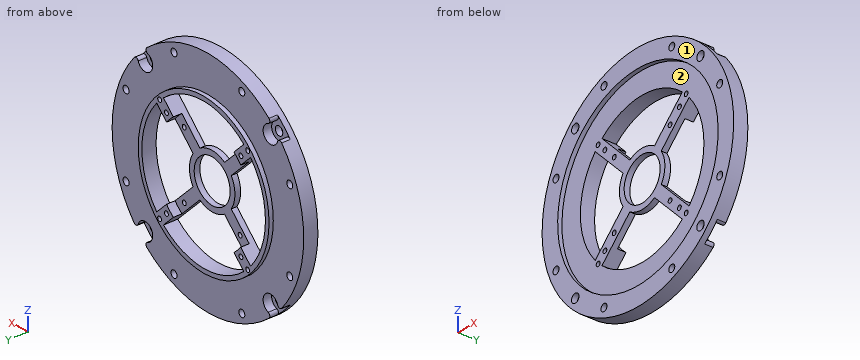
from build123d import *

# Parameters (mm, degrees)
SKETCH_1_R                       = 40
EXTRUDE_1_DEPTH                  = 5
CUT_EXTRUDE_1_DEPTH              = 57.789083458
CUT_EXTRUDE_1_DEPTH_BACK         = 1.5
SKETCH_2_R                       = 33.5
SKETCH_7_R                       = 27.3
EXTRUDE_3_DEPTH                  = 1.5
SKETCH_3_R                       = 25.8
CUT_EXTRUDE_2_DEPTH              = 57.940758688
EXTRUDE_2_DEPTH                  = 5
CUT_EXTRUDE_3_DEPTH              = 57.789083458
CUT_EXTRUDE_3_DEPTH_BACK         = 4
SKETCH_5_R                       = 7.515
CUT_EXTRUDE_4_DEPTH              = 57.835288334
CUT_EXTRUDE_4_DEPTH_BACK         = 57.835288334
SKETCH_6_R                       = 6.5
SKETCH_8_R                       = 20
SKETCH_8_R_2                     = 4.5
CUT_EXTRUDE_5_DEPTH              = 3
HOLE_WIZARD_M2_1_D               = 1.6
HOLE_WIZARD_M2_6_D               = 1.6
HOLE_WIZARD_M3_1_OUTLINE_R       = 1.25
HOLE_WIZARD_M3_1_DEPTH           = 5
SKETCH_25_R                      = 3.1
CUT_EXTRUDE_7_DEPTH              = 3
SKETCH_26_R                      = 1.55
CUT_EXTRUDE_8_DEPTH              = 57.747246629
FILLET_1_R                       = 1
PATTERN_CIRCULAR_1_COUNT         = 4
FILLET_1_OF_PATTERN_CIRCULAR_1_R = 1


# Read off the part's stored shape, not the designer's step: M3 螺纹孔1
with BuildPart() as part:
    # 草图1 → 凸台-拉伸1 (new body)
    with BuildSketch(Plane(origin=(0, 0, 0), x_dir=(1, 0, 0), z_dir=(0, 1, 0))):
        with Locations(Location((0, 0, 0), (0, 0, 270))):
            Circle(SKETCH_1_R)
    extrude(amount=EXTRUDE_1_DEPTH)

    # 草图2 → 切除-拉伸1 (cut, two sides: drawn at the far end of the back side and taken through both)
    with BuildSketch(Plane.XZ.offset(-CUT_EXTRUDE_1_DEPTH_BACK)):
        with Locations(Location((0, 0, 0), (0, 0, 90))):
            Circle(SKETCH_2_R)
    extrude(amount=CUT_EXTRUDE_1_DEPTH + CUT_EXTRUDE_1_DEPTH_BACK, mode=Mode.SUBTRACT)

    # 草图7 → 凸台-拉伸3 (add)
    with BuildSketch(Plane(origin=(0, 5, 0), x_dir=(1, 0, 0), z_dir=(0, 1, 0))):
        with Locations(Location((0, 0, 0), (0, 0, 270))):
            Circle(SKETCH_7_R)
    extrude(amount=EXTRUDE_3_DEPTH)

    # 草图3 → 切除-拉伸2 (cut, through all)
    with BuildSketch(Plane(origin=(0, 6.5, 0), x_dir=(1, 0, 0), z_dir=(0, 1, 0))):
        with Locations(Location((0, 0, 0), (0, 0, 270))):
            Circle(SKETCH_3_R)
    extrude(amount=-CUT_EXTRUDE_2_DEPTH, mode=Mode.SUBTRACT)

    # 草图4 → 凸台-拉伸2 (add)
    with BuildSketch(Plane.XZ.offset(-1.5)):
        with BuildLine():
            Line((-19.657568517, 16.829141392), (-7.981176331, 5.152749206))
            ThreePointArc((-7.981176331, 5.152749206), (-9.5, 0), (-7.981176331, -5.152749206))
            Line((-7.981176331, -5.152749206), (-19.657568517, -16.829141392))
            Line((-19.657568517, -16.829141392), (-16.829141392, -19.657568517))
            Line((-16.829141392, -19.657568517), (-5.152749206, -7.981176331))
            ThreePointArc((-5.152749206, -7.981176331), (0, -9.5), (5.152749206, -7.981176331))
            Line((5.152749206, -7.981176331), (16.829141392, -19.657568517))
            Line((16.829141392, -19.657568517), (19.657568517, -16.829141392))
            Line((19.657568517, -16.829141392), (7.981176331, -5.152749206))
            ThreePointArc((7.981176331, -5.152749206), (9.5, 0), (7.981176331, 5.152749206))
            Line((7.981176331, 5.152749206), (19.657568517, 16.829141392))
            Line((19.657568517, 16.829141392), (16.829141392, 19.657568517))
            Line((16.829141392, 19.657568517), (5.152749206, 7.981176331))
            ThreePointArc((5.152749206, 7.981176331), (0, 9.5), (-5.152749206, 7.981176331))
            Line((-5.152749206, 7.981176331), (-16.829141392, 19.657568517))
            Line((-16.829141392, 19.657568517), (-19.657568517, 16.829141392))
        make_face()
    extrude(amount=-EXTRUDE_2_DEPTH)

    # 草图5 → 切除-拉伸3 (cut, two sides: drawn at the far end of the back side and taken through both)
    with BuildSketch(Plane.XZ.offset(-1.5).offset(-CUT_EXTRUDE_3_DEPTH_BACK)):
        with Locations(Location((0, 0, 0), (0, 0, 270))):
            Circle(SKETCH_5_R)
    extrude(amount=CUT_EXTRUDE_3_DEPTH + CUT_EXTRUDE_3_DEPTH_BACK, mode=Mode.SUBTRACT)

    # 草图6 → 切除-拉伸4 (cut, two sides: drawn at the far end of the back side and taken through both)
    with BuildSketch(Plane.XZ.offset(-5.5).offset(-CUT_EXTRUDE_4_DEPTH_BACK)):
        with Locations(Location((0, 0, 0), (0, 0, 270))):
            Circle(SKETCH_6_R)
    extrude(amount=CUT_EXTRUDE_4_DEPTH + CUT_EXTRUDE_4_DEPTH_BACK, mode=Mode.SUBTRACT)

    # 草图8 → 切除-拉伸5 (cut)
    with BuildSketch(Plane(origin=(0, 6.5, 0), x_dir=(1, 0, 0), z_dir=(0, 1, 0))):
        Circle(SKETCH_8_R)
        Circle(SKETCH_8_R_2, mode=Mode.SUBTRACT)
    extrude(amount=-CUT_EXTRUDE_5_DEPTH, mode=Mode.SUBTRACT)

    # M2 螺纹孔1 (through all)
    with Locations(Plane(origin=(0, 3.5, 0), x_dir=(1, 0, 0), z_dir=(0, 1, 0))):
        with Locations((0, 0), (-11.66726189, 11.66726189), (11.66726189, 11.66726189), (11.66726189, -11.66726189), (-11.66726189, -11.66726189)):
            Hole(HOLE_WIZARD_M2_1_D / 2)

    # M2 螺纹孔6 (through all)
    with Locations(Plane(origin=(0, 6.5, 0), x_dir=(1, 0, 0), z_dir=(0, 1, 0))):
        with Locations((15.556349186, 15.556349186), (0, 0), (-15.556349186, 15.556349186), (-15.556349186, -15.556349186), (15.556349186, -15.556349186), (-18.384776311, 18.384776311), (18.384776311, 18.384776311), (18.384776311, -18.384776311), (-18.384776311, -18.384776311)):
            Hole(HOLE_WIZARD_M2_6_D / 2)

    # M3 螺纹孔1 outline → M3 螺纹孔1 (cut)
    with BuildSketch(Plane(origin=(0, 0, 0), x_dir=(1, 0, 0), z_dir=(0, 1, 0))):
        with Locations((34.183542703, 14.159286998)):
            Circle(HOLE_WIZARD_M3_1_OUTLINE_R)
        with Locations((34.183542703, -14.159286998)):
            Circle(HOLE_WIZARD_M3_1_OUTLINE_R)
        with Locations((14.159286998, -34.183542703)):
            Circle(HOLE_WIZARD_M3_1_OUTLINE_R)
        with Locations((-14.159286998, -34.183542703)):
            Circle(HOLE_WIZARD_M3_1_OUTLINE_R)
        with Locations((-34.183542703, -14.159286998)):
            Circle(HOLE_WIZARD_M3_1_OUTLINE_R)
        with Locations((-34.183542703, 14.159286998)):
            Circle(HOLE_WIZARD_M3_1_OUTLINE_R)
        with Locations((-14.159286998, 34.183542703)):
            Circle(HOLE_WIZARD_M3_1_OUTLINE_R)
        with Locations((14.159286998, 34.183542703)):
            Circle(HOLE_WIZARD_M3_1_OUTLINE_R)
    extrude(amount=HOLE_WIZARD_M3_1_DEPTH, mode=Mode.SUBTRACT)

    # 草图25 → 切除-拉伸7 (cut)
    with BuildSketch(Plane(origin=(0, 5, 0), x_dir=(1, 0, 0), z_dir=(0, 1, 0))):
        with Locations((-26.162950904, -26.162950904)):
            Circle(SKETCH_25_R)
    cut_extrude_7 = extrude(amount=-CUT_EXTRUDE_7_DEPTH, mode=Mode.SUBTRACT)

    # 草图26 → 切除-拉伸8 (cut, through all)
    with BuildSketch(Plane(origin=(0, 2, 0), x_dir=(1, 0, 0), z_dir=(0, 1, 0))):
        with Locations(Location((-26.162950904, -26.162950904, 0), (0, 0, 270))):
            Circle(SKETCH_26_R)
    cut_extrude_8 = extrude(amount=-CUT_EXTRUDE_8_DEPTH, mode=Mode.SUBTRACT)

    # 圆角1
    fillet_1_edges = [part.edges().sort_by_distance(p)[0] for p in [
        (-28.852633786, 3.5, 27.704251003),
        (-27.704251003, 3.5, 28.852633786),
    ]]
    fillet(fillet_1_edges, radius=FILLET_1_R)

    # 阵列(圆周)1: 切除-拉伸7, 切除-拉伸8 ×4 about axis
    pattern_circular_1_axis = Axis((0, 0, 0), (0, 1, 0))
    add([cut_extrude_7.rotate(pattern_circular_1_axis, i * 360 / PATTERN_CIRCULAR_1_COUNT) for i in range(1, PATTERN_CIRCULAR_1_COUNT)], mode=Mode.SUBTRACT)
    add([cut_extrude_8.rotate(pattern_circular_1_axis, i * 360 / PATTERN_CIRCULAR_1_COUNT) for i in range(1, PATTERN_CIRCULAR_1_COUNT)], mode=Mode.SUBTRACT)

    # 圆角1 of 阵列(圆周)1
    fillet_1_of_pattern_circular_1_edges = [part.edges().sort_by_distance(p)[0] for p in [
        (27.704251003, 3.5, 28.852633786),
        (28.852633786, 3.5, 27.704251003),
        (28.852633786, 3.5, -27.704251003),
        (27.704251003, 3.5, -28.852633786),
        (-27.704251003, 3.5, -28.852633786),
        (-28.852633786, 3.5, -27.704251003),
    ]]
    fillet(fillet_1_of_pattern_circular_1_edges, radius=FILLET_1_OF_PATTERN_CIRCULAR_1_R)


solid = part.part
Could you check a few things on this model? Use its own coordinates, in mm. Face numbers are marked on the shaded views. Give positions to 0.01 mm unless a question says otherwise; leave off trailing zeros. Order: outer loops, then holes, each group sorted by start corner. A loop starts at its lowest first (then second) coordinate and runs counter-clockwise, first axis right, second up. Notation, with made-up numbers: (10.5, 81.5) -> (19.5, 81.5) arc R19 cw to (19.5, 103.5) -> close; hole circle Ø1 at (28, -31.75). An arc over 180 degrees is marked (long way). Answer in a Markdown table with one row per item. Add a question column.
Item 1: We'd pull the mould along X, two halves only. Please class the marked faces 1 and 2: pulls with the +X half, pulls with the -X half, needs draft (parallel to the pull), parting line crosses it, or undercut.
Item 2: Imagine slicing it at D-D (x = -32). List the corners of the cut face in (y, z) for me.
Item 3: Imagine slicing it at B-B (z = 21). List the corners of the cut face in (x, y) for me.
Item 4: Please list where these lines run through material, in increasing order: probe 1 along Z at (x, y) = (6, 3); probe 2 along X at (y, z) = (3.25, -18); probe 3 along X at (y, z) = (2.5, 4.5).
Item 5: I'm going to push flat-ended pins straight in: P1, Ø1, axis at y = 2, z = 1.5, coming from the +X side; P2, Ø1.8, axis at x = -18.38, z = -18.38, coming from the -Y side; P3, Ø4, axis at x = 5, z = -3.5, coming from the +Y side; P4, Ø2.5, axis at x = 18.38, z = 18.38, coming from the +Y side. Where does each tip first touch, or does it pass through?
Item 6: Imagine slicing it at A-A (x = 0). List the corners of the cut face in (y, z) for me (3 decimals).
Item 7: Imagine slicing it at C-C (z = 0). List the corners of the cut face in (x, y) for me (3 decimals), and give its area (3 significant figures).
Result:
| question | item | result |
|---|---|---|
| 1 | face 1 | needs draft |
| 1 | face 2 | undercut |
| 2 | outline | (0, -24) -> (5, -24) -> (5, 24) -> (0, 24) -> (0, 9.91) -> (1.5, 9.91) -> (1.5, -9.91) -> (0, -9.91) -> close |
| 3 | outline | (-34.04, 0) -> (-26.1, 0) -> (-26.1, 1.5) -> (-14.99, 1.5) -> (-14.99, 6.5) -> (-17.44, 6.5) -> (-17.44, 5) -> (-34.04, 5) -> close; (14.99, 1.5) -> (26.1, 1.5) -> (26.1, 0) -> (34.04, 0) -> (34.04, 5) -> (17.44, 5) -> (17.44, 6.5) -> (14.99, 6.5) -> close |
| 4 | probe 1 | -39.55 to -25.09, -8.83 to -4.52, 4.52 to 8.83, 25.09 to 39.55 |
| 4 | probe 2 | -35.72 to -19.09, -17.68 to -15.17, 15.17 to 17.68, 19.09 to 35.72 |
| 4 | probe 3 | -39.75 to -25.4, -8.37 to -6.02, 6.02 to 8.37, 25.4 to 39.75 |
| 5 | P1 | x = 39.99 |
| 5 | P2 | y = 1.5 |
| 5 | P3 | y = 3.5 |
| 5 | P4 | y = 6.5 |
| 6 | outline | (0, -40) -> (5, -40) -> (5, -27.3) -> (6.5, -27.3) -> (6.5, -25.8) -> (1.5, -25.8) -> (1.5, -33.5) -> (0, -33.5) -> close; (0, 33.5) -> (1.5, 33.5) -> (1.5, 25.8) -> (6.5, 25.8) -> (6.5, 27.3) -> (5, 27.3) -> (5, 40) -> (0, 40) -> close; (1.5, -9.5) -> (3.5, -9.5) -> (3.5, -7.515) -> (1.5, -7.515) -> close; (1.5, 7.515) -> (3.5, 7.515) -> (3.5, 9.5) -> (1.5, 9.5) -> close |
| 7 | outline | (-40, 0) -> (-33.5, 0) -> (-33.5, 1.5) -> (-25.8, 1.5) -> (-25.8, 6.5) -> (-27.3, 6.5) -> (-27.3, 5) -> (-40, 5) -> close; (-9.5, 1.5) -> (-7.515, 1.5) -> (-7.515, 3.5) -> (-9.5, 3.5) -> close; (7.515, 1.5) -> (9.5, 1.5) -> (9.5, 3.5) -> (7.515, 3.5) -> close; (25.8, 1.5) -> (33.5, 1.5) -> (33.5, 0) -> (40, 0) -> (40, 5) -> (27.3, 5) -> (27.3, 6.5) -> (25.8, 6.5) -> close |
| 7 | area | 131 mm2 |
